Here's how the part is built. I have some questions about the finished solid (model axes, mm). Face numbers are marked on the shaded views. A direction names the side the tool comes from. Coordinates: 2 decimals unless noted, no trailing zeros. Write each loop counter-clockwise with the first axis right and the second up, starting at its lowest first coordinate (ties: lowest second). Pieces come first, ordered by that corner, then holes.
from build123d import *

# Parameters (mm, degrees)
ESQUISSE1_R             = 1.6
BOSS_EXTRU_1_DEPTH      = 15.5
ESQUISSE2_W             = 88.683684882
ESQUISSE2_H             = 17.311737923
ENL_V_MAT_EXTRU_1_DEPTH = 4
ENL_V_START             = -15.5
ESQUISSE2_2_W           = 88.683684882
ESQUISSE2_2_H           = 17.311737923
ENL_V_MAT_EXTRU_2_DEPTH = 2
ESQUISSE3_W             = 40.5
ESQUISSE3_H             = 10.25
ENL_V_MAT_EXTRU_3_DEPTH = 39.399218742
ESQUISSE4_R             = 1.25
ENL_V_MAT_EXTRU_4_DEPTH = 38.369773882
ESQUISSE5_R             = 3.5
ENL_V_MAT_EXTRU_5_DEPTH = 37.558172821
BOSS_EXTRU_2_START      = -1.75
BOSS_EXTRU_2_DEPTH      = 1.75
BOSS_EXTRU_3_START      = -15.5
BOSS_EXTRU_3_DEPTH      = 1.58
CONG_1_R                = 1


with BuildPart() as part:
    # Esquisse1 → Boss.-Extru.1 (new body)
    with BuildSketch(Plane(origin=(0, 0, 0), x_dir=(1, 0, 0), z_dir=(0, 1, 0))):
        with BuildLine():
            Line((-22.5, 5.5), (22.5, 5.5))
            ThreePointArc((22.5, 5.5), (24.974873734, 4.474873734), (26, 2))
            Line((26, 2), (26, 0))
            ThreePointArc((26, 0), (29, -3), (32, 0))
            ThreePointArc((32, 0), (28.631727984, 8.131727984), (20.5, 11.5))
            Line((20.5, 11.5), (-20.5, 11.5))
            ThreePointArc((-20.5, 11.5), (-28.631727984, 8.131727984), (-32, 0))
            ThreePointArc((-32, 0), (-29, -3), (-26, 0))
            Line((-26, 0), (-26, 2))
            ThreePointArc((-26, 2), (-24.974873734, 4.474873734), (-22.5, 5.5))
        make_face()
        with Locations(Location((-29, 0, 0), (0, 0, 270))):
            Circle(ESQUISSE1_R, mode=Mode.SUBTRACT)
        with Locations(Location((29, 0, 0), (0, 0, 270))):
            Circle(ESQUISSE1_R, mode=Mode.SUBTRACT)
    extrude(amount=BOSS_EXTRU_1_DEPTH)

    # Esquisse2 → Enlèv. mat.-Extru.1 (cut)
    with BuildSketch(Plane(origin=(0, 15.5, 0), x_dir=(1, 0, 0), z_dir=(0, 1, 0))):
        with Locations((-5.127432495, -5.155868962)):
            Rectangle(ESQUISSE2_W, ESQUISSE2_H)
    extrude(amount=-ENL_V_MAT_EXTRU_1_DEPTH, mode=Mode.SUBTRACT)

    # Esquisse2<2> → Enlèv. mat.-Extru.2 (cut)
    with BuildSketch(Plane(origin=(0, 15.5, 0), x_dir=(1, 0, 0), z_dir=(0, 1, 0)).offset(ENL_V_START)):
        with Locations((-5.127432495, -5.155868962)):
            Rectangle(ESQUISSE2_2_W, ESQUISSE2_2_H)
    extrude(amount=ENL_V_MAT_EXTRU_2_DEPTH, mode=Mode.SUBTRACT)

    # Esquisse3 → Enlèv. mat.-Extru.3 (cut, through all)
    with BuildSketch(Plane(origin=(0, 0, -11.5), x_dir=(-1, 0, 0), z_dir=(0, 0, -1))):
        with Locations((-2.440596151, 8.625)):
            Rectangle(ESQUISSE3_W, ESQUISSE3_H)
    extrude(amount=-ENL_V_MAT_EXTRU_3_DEPTH, mode=Mode.SUBTRACT)

    # Esquisse4 → Enlèv. mat.-Extru.4 (cut, through all)
    with BuildSketch(Plane(origin=(0, 15.5, 0), x_dir=(1, 0, 0), z_dir=(0, 1, 0))):
        with Locations(Location((19.940596151, 8, 0), (0, 0, 270))):
            Circle(ESQUISSE4_R)
        with Locations(Location((-15.059403849, 8, 0), (0, 0, 270))):
            Circle(ESQUISSE4_R)
    extrude(amount=-ENL_V_MAT_EXTRU_4_DEPTH, mode=Mode.SUBTRACT)

    # Esquisse5 → Enlèv. mat.-Extru.5 (cut, through all)
    with BuildSketch(Plane.XY.offset(-5.5)):
        with Locations((-21.5, 4.9)):
            Circle(ESQUISSE5_R)
        with BuildLine():
            Line((13.351466812, 5.58), (24, 5.58))
            ThreePointArc((24, 5.58), (26, 3.58), (24, 1.58))
            Line((24, 1.58), (13.351466812, 1.58))
            ThreePointArc((13.351466812, 1.58), (11.351466812, 3.58), (13.351466812, 5.58))
        make_face()
    extrude(amount=ENL_V_MAT_EXTRU_5_DEPTH, mode=Mode.SUBTRACT)

    # Esquisse6 → Boss.-Extru.2 (add)
    with BuildSketch(Plane(origin=(0, 15.5, 0), x_dir=(1, 0, 0), z_dir=(0, 1, 0)).offset(BOSS_EXTRU_2_START)):
        with BuildLine():
            Line((-22.5, 5.5), (22.5, 5.5))
            ThreePointArc((22.5, 5.5), (24.370828693, 4.958039892), (25.66227766, 3.5))
            Line((25.66227766, 3.5), (-25.66227766, 3.5))
            ThreePointArc((-25.66227766, 3.5), (-24.370828693, 4.958039892), (-22.5, 5.5))
        make_face()
    extrude(amount=BOSS_EXTRU_2_DEPTH)

    # Esquisse6<2> → Boss.-Extru.3 (add)
    with BuildSketch(Plane(origin=(0, 15.5, 0), x_dir=(1, 0, 0), z_dir=(0, 1, 0)).offset(BOSS_EXTRU_3_START)):
        with BuildLine():
            Line((-22.5, 5.5), (22.5, 5.5))
            ThreePointArc((22.5, 5.5), (24.370828693, 4.958039892), (25.66227766, 3.5))
            Line((25.66227766, 3.5), (-25.66227766, 3.5))
            ThreePointArc((-25.66227766, 3.5), (-24.370828693, 4.958039892), (-22.5, 5.5))
        make_face()
    extrude(amount=BOSS_EXTRU_3_DEPTH)

    # Congé1
    cong_1_edges = [part.edges().sort_by_distance(p)[0] for p in [
        (-31.45445115, 13.5, -3.5),
        (31.45445115, 13.5, -3.5),
        (-31.45445115, 1, -3.5),
        (31.45445115, 1, -3.5),
    ]]
    fillet(cong_1_edges, radius=CONG_1_R)


solid = part.part
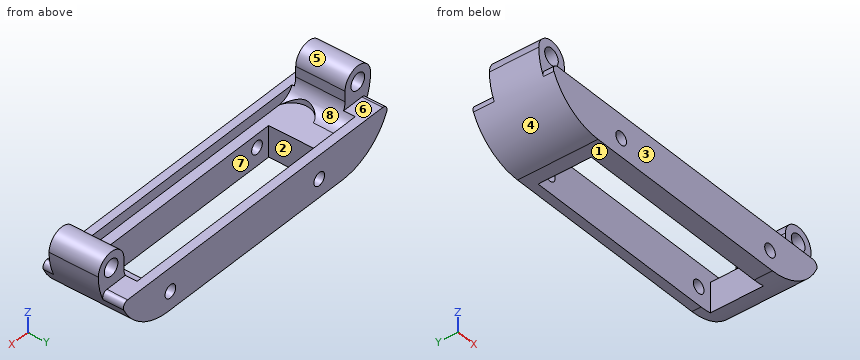
1. I want a section at D-D (y = 6.75). List the corners of the cut face in (x, z) for me.
2. For pin 1 Ø5 at (x, z) = (29, 0) entering from +Y; pin 2 Ø5 at (y, z) = (6.5, -3) entering from +X; pin 3 Ø1.5 at (x, z) = (19.94, -8) entering from +Y; pin 4 Ø5 at (y, z) = (6, -4.5) entering from -X, each with a flat end and sliding along its axis, tell me the tip position at first contact or that it passes through.
3. I want a section at B-B (x = -7.5). List the corners of the cut face in (y, z) for me, then the cut area to 3 significant figures.
4. I want a section at A-A (y = 9.25). List the corners of the cut face in (x, z) for me, then the cut area to 3 significant figures.
5. I want a section at C-C (z = -7.5). List the corners of the cut face in (x, y) for me.
6. On a 3-axis mill with a long thin cutter (end or side, diameter ignored), from which of +Z, -Z, +X, -X, +Y, -Y can I reach the whole of each face in a straight line? I mean the marked faces 4, 5, 6, 7 and 8. Say none if no direction works.
7. Thinking about a two-plate mould opening in Y: for the marked faces 1, 2 and 3, which applies, pulls with the +Y half, pulls with the -Y half, needs draft (parallel to the pull), parting line crosses it, or undercut?
8. If I drill on line 1 (X direction, y = 9.75, z = 0); line 2 (Y direction, x = -2.5, z = -7.5); line 3 (X direction, y = 2.25, z = 1), over which ranges is the centre line in solid material (lowest first)?
Response values:
1. outline: (-32, 0) arc R11.5 ccw to (-20.5, -11.5) - (-17.81, -11.5) - (-17.81, -5.5) - (-24.47, -5.5) - (-24.47, -4.89) arc R3.5 cw to (-26, -2) - (-26, 0) arc R3 ccw to start; (22.69, -11.29) arc R11.5 ccw to (32, 0) arc R3 ccw to (26, 0) - (26, -2) arc R3.5 cw to (22.69, -5.49) - close; hole circle Ø3.2 at (-29, 0); hole circle Ø3.2 at (29, 0)
2. pin 1: stops at y = 11.5
2. pin 2: stops at x = 31.99
2. pin 3: passes through
2. pin 4: stops at x = -31.82
3. outline: (0, -11.5) - (3.5, -11.5) - (3.5, -5.5) - (1.58, -5.5) - (1.58, -3.5) - (0, -3.5) - close; (13.75, -11.5) - (15.5, -11.5) - (15.5, -3.5) - (13.75, -3.5) - close
3. area: 38.2 mm2
4. outline: (-32, 0) arc R11.5 ccw to (-20.5, -11.5) - (-17.81, -11.5) - (-17.81, -5.5) - (-22.5, -5.5) arc R3.5 cw to (-26, -2) - (-26, 0) arc R3 ccw to start; (22.69, -11.29) arc R11.5 ccw to (32, 0) arc R3 ccw to (26, 0) - (26, -2) arc R3.5 cw to (22.69, -5.49) - close; hole circle Ø3.2 at (-29, 0); hole circle Ø3.2 at (29, 0)
4. area: 168 mm2
5. outline: (-29.22, 0) - (-16.21, 0) - (-16.21, 3.5) - (-17.81, 3.5) - (-17.81, 13.75) - (-16.21, 13.75) - (-16.21, 15.5) - (-29.22, 15.5) - close; (-13.91, 0) - (18.79, 0) - (18.79, 3.5) - (-13.91, 3.5) - close; (-13.91, 13.75) - (18.79, 13.75) - (18.79, 15.5) - (-13.91, 15.5) - close; (21.09, 0) - (29.22, 0) - (29.22, 15.5) - (21.09, 15.5) - (21.09, 13.75) - (22.69, 13.75) - (22.69, 3.5) - (21.09, 3.5) - close
6. face 4: -Z, -X, +Y, -Y
6. face 5: +Z, +Y, -Y
6. face 6: +Z, +X, -X, +Y
6. face 7: +Z, -Z
6. face 8: +Z
7. face 1: needs draft
7. face 2: undercut
7. face 3: pulls with the -Y half
8. line 1: x = -32 to -30.6, -27.4 to -26, 26 to 27.4, 30.6 to 32
8. line 2: y = 0 to 3.5, 13.75 to 15.5
8. line 3: x = -31.83 to -30.25, -27.75 to -26.17, 26.17 to 27.75, 30.25 to 31.83
